Source: CAD feature listing. Evaluate the final solid. Frame: model axes, mm. A direction names the side the tool comes from. Give positions to 0.01 mm unless a question says otherwise; leave off trailing zeros. Order: outer loops, then holes, each group sorted by start corner. A loop starts at its lowest first (then second) coordinate and runs counter-clockwise, first axis right, second up.
from build123d import *

# Parameters (mm, degrees)
CYLINDER001_R           = 6
CYLINDER001_DEPTH       = 1300
CYLINDER001_PITCH_ANGLE = 90
CYLINDER002_R           = 6
CYLINDER002_DEPTH       = 900
CYLINDER002_ROLL_ANGLE  = -90
BOX003_W                = 80
BOX003_H                = 80
BOX003_DEPTH            = 750
BOX002_W                = 80
BOX002_H                = 80
BOX002_DEPTH            = 750


with BuildPart() as cylinder001:
    # Cylinder001 → Cylinder001 (new body)
    with BuildSketch(Plane.XY):
        Circle(CYLINDER001_R)
    extrude(amount=CYLINDER001_DEPTH)


with BuildPart() as cylinder001_1:
    # Cylinder001 pitch: moved
    add(cylinder001.part.rotate(Axis((0, 0, 0), (0, 1, 0)), CYLINDER001_PITCH_ANGLE))


with BuildPart() as cylinder001_2:
    # Cylinder001 placement: moved
    add(cylinder001_1.part.moved(Location((-10, 840, 720))))


with BuildPart() as cylinder002:
    # Cylinder002 → Cylinder002 (new body)
    with BuildSketch(Plane.XY):
        Circle(CYLINDER002_R)
    extrude(amount=CYLINDER002_DEPTH)


with BuildPart() as cylinder002_1:
    # Cylinder002 roll: moved
    add(cylinder002.part.rotate(Axis((0, 0, 0), (1, 0, 0)), CYLINDER002_ROLL_ANGLE))


with BuildPart() as cylinder002_2:
    # Cylinder002 placement: moved
    add(cylinder002_1.part.moved(Location((40, -10, 700))))


with BuildPart() as cube003:
    # Box003 → Box003 (new body)
    with BuildSketch(Plane(origin=(8, 792, 0), x_dir=(1, 0, 0), z_dir=(0, 0, 1))):
        with Locations((40, 40)):
            Rectangle(BOX003_W, BOX003_H)
    extrude(amount=BOX003_DEPTH)


with BuildPart() as cut008:
    # Box002 → Box002 (new body)
    with BuildSketch(Plane(origin=(0, 800, 0), x_dir=(1, 0, 0), z_dir=(0, 0, 1))):
        with Locations((40, 40)):
            Rectangle(BOX002_W, BOX002_H)
    extrude(amount=BOX002_DEPTH)

    # Cut001: cut Cube003
    add(cube003.part, mode=Mode.SUBTRACT)

    # Cut007: cut Cylinder002
    add(cylinder002_2.part, mode=Mode.SUBTRACT)

    # Cut008: cut Cylinder001
    add(cylinder001_2.part, mode=Mode.SUBTRACT)


solid = cut008.part
1) First-contact query: pin 1 Ø1 at (x, z) = (43, 137.5) entering from -Y. Flat tip, straight axial feed; report the tip coordinate or a pass-through.
Checks:
pin 1: stops at y = 872
2) Section query C-C on x = 54. Output: boundary loops of the cut face in (y, z).
Checks:
outline: (872, 0) - (880, 0) - (880, 750) - (872, 750) - close
3) Pull-direction query (X, two-part tool) for faces 1 (the face through (8, 835, 370)), 2 (the face through (39.22, 875.94, 694.05)), 3 (the face through (0, 839, 370)), 4 (the face through (3.94, 837.7, 714.46)); classes: +X half, -X half, draft (parallel to the pull), parting line (faces both ways), or undercut.
Checks:
face 1: +X half
face 2: undercut
face 3: -X half
face 4: draft
4) Section query A-A on z = 189.5. Output: boundary loops of the cut face in (x, y), and give its area (3 significant figures).
Checks:
outline: (0, 800) - (8, 800) - (8, 872) - (80, 872) - (80, 880) - (0, 880) - close
area: 1,220 mm2
5) Ray query, L1, parallel to Z at x = 40, y = 874; L2, parallel to Z at x = 2, y = 840; L3, parallel to Y at x = 2, z = 720. Return the intervals inside material, ascending.
Checks:
L1: z = 0 to 694, 706 to 750
L2: z = 0 to 714, 726 to 750
L3: y = 800 to 834, 846 to 880
6) Section query B-B on y = 821.5. Output: boundary loops of the cut face in (x, z), and give its area (3 significant figures).
Checks:
outline: (0, 0) - (8, 0) - (8, 750) - (0, 750) - close
area: 6,000 mm2
7) Reachability of faces 5 (the face through (39, 880, 370)), 6 (the face through (43, 872, 370)) from +Z, -Z, +X, -X, +Y, -Y: full face, straight path, thin tool, end or side. Return the list, or none.
Checks:
face 5: +Z, -Z, +X, -X, +Y
face 6: +Z, -Z, +X, -Y
